from build123d import *

# Parameters (mm, degrees)
F1_DEPTH = 12.5
F3_R     = 4.25
F4_DEPTH = 25.4
F2_R     = 4.25
F5_DEPTH = 54.356
F6_W     = 12.369135
F6_H     = 5.527861
F7_DEPTH = 25.4


with BuildPart() as f1:
    # F0 (on Front) → F1 (new body)
    with BuildSketch(Plane.XZ):
        with BuildLine():
            Line((-2.776492, 16.536297), (-32.776492, 16.536297))
            Line((-32.776492, 16.536297), (-60.96727, 6.275693))
            Line((-60.96727, 6.275693), (-75.96727, 32.256455))
            Line((-75.96727, 32.256455), (-88.46727, 32.256455))
            Line((-88.46727, 32.256455), (-71.295553, 2.514168))
            ThreePointArc((-71.295553, 2.514168), (-64.640686, -3.069928), (-55.953374, -3.069928))
            Line((-55.953374, -3.069928), (-32.461059, 5.480576))
            Line((-32.461059, 5.480576), (-3.091924, 5.480576))
            Line((-3.091924, 5.480576), (20.400391, -3.069928))
            ThreePointArc((20.400391, -3.069928), (29.087703, -3.069928), (35.74257, 2.514168))
            Line((35.74257, 2.514168), (52.914287, 32.256455))
            Line((52.914287, 32.256455), (40.414287, 32.256455))
            Line((40.414287, 32.256455), (25.414287, 6.275693))
            Line((25.414287, 6.275693), (-2.776492, 16.536297))
        make_face()
    extrude(amount=F1_DEPTH)

    # F3 (on face) → F4 (cut)
    with BuildSketch(Plane.XY.offset(32.256455)):
        with Locations((-82.21727, -6.25)):
            Circle(F3_R)
    extrude(amount=-F4_DEPTH, mode=Mode.SUBTRACT)

    # F2 (on face) → F5 (cut)
    with BuildSketch(Plane.XY.offset(32.256455)):
        with Locations((46.664287, -6.25)):
            Circle(F2_R)
    extrude(amount=-F5_DEPTH, mode=Mode.SUBTRACT)

    # F6 (on face) → F7 (cut)
    with BuildSketch(Plane.XZ.offset(12.5)):
        with Locations((-17.776491, 8.244506)):
            Rectangle(F6_W, F6_H)
    extrude(amount=-F7_DEPTH, mode=Mode.SUBTRACT)


solid = f1.part
The model under review builds one solid part; all positions refer to its coordinate system, in mm. A direction names the side the tool comes from. Give positions to 0.01 mm unless a question says otherwise; leave off trailing zeros. Order: outer loops, then holes, each group sorted by start corner. A loop starts at its lowest first (then second) coordinate and runs counter-clockwise, first axis right, second up. Notation, with made-up numbers: M 22,78.5 L 74,78.5 A15 cw 74,102.5 Z; hole C 35,83 d5. An arc over 180 degrees is marked long. Answer in a Markdown table with one row per item. Add a question column.
1. Add section C-C on z = 8.5. State the section outline as (x, y) points, plus the area to 3 significant figures.
2. Add section B-B on z = 19. State the section outline as (x, y) points.
3. To check wall thickness, follow line 1 along Z through (x, y) = (-14, -9.5); line 2 along X through (y, z) = (-1.5, 27); line 3 along X through (y, z) = (-6.25, 19). State the ranges of each line that lie inside material, in increasing order.
4. Mouldability with a two-part tool opening along X and no side actions: class faces 1 (the flat face through (-78.1, -4.8, 14.3)), 2 (the flat face through (-18, 0, 13)), 3 (the cylindrical face through (29, -6.2, -3.1)) as released by +X, released by -X, zero draft, split by the parting line, or undercut.
5. Add section D-D on x = -38. State the section outline as (y, z) points, plus the area to 3 significant figures.
6. Machinability: for faces 4 (the flat face through (-18, -6, 16.536)), 5 (the flat face through (-18, -6, 11.008)), 6 (the flat face through (42.3, -6.16, 13.87)), which of the approach directions +Z, -Z, +X, -X, +Y, -Y give a long, thin tool a straight path to every point of the face, cutting with its end or side? Answer none if there is none.
7. For pin 1 Ø2 at (x, y) = (19, -10.5) entering from -Z; pin 2 Ø7 at (x, y) = (-27, -6.5) entering from -Z; pin 3 Ø5 at (y, z) = (-11, 16) entering from -X (3 decimals), all flat-tipped, find the tip position at first contact; note any pin that passes through.
8. Add section A-A on y = -7.5. State the section outline as (x, z) points, plus the area to 3 significant figures.
The answers:
| question | item | result |
|---|---|---|
| 1 | outline | M -74.75,-12.5 L -62.25,-12.5 L -62.25,0 L -74.75,0 Z; M -54.86,-12.5 L -23.96,-12.5 L -23.96,0 L -54.86,0 Z; M -11.59,-12.5 L 19.3,-12.5 L 19.3,0 L -11.59,0 Z; M 26.7,-12.5 L 39.2,-12.5 L 39.2,0 L 26.7,0 Z |
| 1 | area | 1,080 mm2 |
| 2 | outline | M -80.81,-12.5 L -68.31,-12.5 L -68.31,0 L -80.81,0 L -80.81,-2.24 A4.25 cw -80.81,-10.26 Z; M 32.76,-12.5 L 45.26,-12.5 L 45.26,-10.26 A4.25 cw 45.26,-2.24 L 45.26,0 L 32.76,0 Z |
| 3 | line 1 | 11.01 to 16.54 |
| 3 | line 2 | -85.43 to -72.93, 37.38 to 49.88 |
| 3 | line 3 | -77.97 to -68.31, 32.76 to 42.41 |
| 4 | face 1 | released by -X |
| 4 | face 2 | zero draft |
| 4 | face 3 | undercut |
| 5 | outline | M -12.5,3.46 L 0,3.46 L 0,14.64 L -12.5,14.64 Z |
| 5 | area | 140 mm2 |
| 6 | face 4 | +Z, +Y, -Y |
| 6 | face 5 | -Z, +Y, -Y |
| 6 | face 6 | -Z, +X, +Y, -Y |
| 7 | pin 1 | z = -2.92 |
| 7 | pin 2 | z = 5.48 |
| 7 | pin 3 | x = -80.525 |
| 8 | outline | M -88.47,32.26 L -86.28,28.47 L -86.28,32.26 Z; M -78.16,14.4 L -71.3,2.51 A12.7 ccw -55.95,-3.07 L -32.46,5.48 L -23.96,5.48 L -23.96,11.01 L -11.59,11.01 L -11.59,5.48 L -3.09,5.48 L 20.4,-3.07 A12.7 ccw 35.74,2.51 L 42.6,14.4 L 42.6,32.26 L 40.41,32.26 L 25.41,6.28 L -2.78,16.54 L -32.78,16.54 L -60.97,6.28 L -75.97,32.26 L -78.16,32.26 Z; M 50.73,28.47 L 52.91,32.26 L 50.73,32.26 Z |
| 8 | area | 1,540 mm2 |
